Source: CAD feature listing. Evaluate the final solid. Frame: model axes, mm. Coordinates: 2 decimals unless noted, no trailing zeros. Order: outer loops, then holes, each group sorted by start corner. A loop starts at its lowest first (then second) coordinate and runs counter-clockwise, first axis right, second up. Notation, with made-up numbers: (-6.75, 36.5) -> (16.25, 36.5) arc R33 ccw to (16.25, 75.5) -> close; hole circle Ø1 at (83, 43). An arc over 180 degrees is marked (long way). Put each result on its own line as item: value.
from build123d import *

# Parameters (mm, degrees)
F0_R      = 57.15
F1_DEPTH  = 2.54
F3_R      = 36.83
F1_FACE_R = 57.15


# Not quite as in the source:
# - the program builds the solid bodies; features that only make, move or delete a surface that nothing else refers to are left out


with BuildPart() as f1:
    # F0 (on Top) → F1 (new body)
    with BuildSketch(Plane.XY):
        Circle(F0_R)
    extrude(amount=F1_DEPTH)

    # F3 (on offset) → F4 section 0
    with BuildSketch(Plane.XY.offset(27.94)):
        Circle(F3_R)
    # F1_face (on face) → F4 section 1
    with BuildSketch(Plane.XY.offset(2.54)):
        Circle(F1_FACE_R)
    loft()

    # F5: F1 across face


with BuildPart() as f1_1:
    add(f1.part)
    add(f1.part.mirror(Plane(origin=(0, 0, 0), x_dir=(1, 0, 0), z_dir=(0, 0, -1))))


solid = f1_1.part
1. Cut plane C-C on z = -5. Output: boundary loops of the cut face in (x, y).
Numbers:
outline: circle Ø110.36 at (0, 0)
2. Cut plane A-A on x = 0. Output: boundary loops of the cut face in (y, z).
Numbers:
outline: (-57.15, -2.54) -> (-36.83, -27.94) -> (36.83, -27.94) -> (57.15, -2.54) -> (57.15, 2.54) -> (36.83, 27.94) -> (-36.83, 27.94) -> (-57.15, 2.54) -> close
3. First-contact query: pin 1 (1.5 mm diameter, centred on x = 3.5, z = 5.5, fed in from -Y); pin 2 (12 mm diameter, centred on x = 20, y = -39.5, fed in from -Z); pin 3 (12 mm diameter, centred on y = 40.5, z = 7.5, fed in from +X). Flat tips, straight axial feed; report the tip coordinate or a pass-through.
Numbers:
pin 1: stops at y = -55.27
pin 2: stops at z = -26.13
pin 3: stops at x = 43.48
4. Cut plane B-B on z = 16.5. Output: boundary loops of the cut face in (x, y), plus the area to 3 significant figures.
Numbers:
outline: circle Ø91.96 at (0, 0)
area: 6,640 mm2
5. Ray query, line 1 along X through (y, z) = (-3.5, 21); line 2 along Z through (x, y) = (47.5, -1.5); line 3 along X through (y, z) = (-2.5, -4). Return the intervals inside material, ascending.
Numbers:
line 1: x = -42.24 to 42.24
line 2: z = -14.57 to 14.57
line 3: x = -55.93 to 55.93
